from build123d import *

# Parameters (mm, degrees)
SKETCH1_R               = 26.25
BOSS_EXTRUDE1_DEPTH     = 1.5
SKETCH2_R               = 17.5
CUT_EXTRUDE1_DEPTH      = 4.5
SKETCH3_R               = 1
CUT_EXTRUDE2_DEPTH      = 2.5
SKETCH5_R               = 1
CUT_EXTRUDE3_DEPTH      = 1.5
BOSS_EXTRUDE4_DEPTH     = 1.5
CUT_EXTRUDE4_DEPTH      = 10
CUT_EXTRUDE4_DEPTH_BACK = 1.5
SKETCH7_R               = 1.75
SKETCH12_R              = 2.5
BOSS_EXTRUDE6_DEPTH     = 1.5
CUT_EXTRUDE5_START      = 1.5
SKETCH13_R              = 1.75
CUT_EXTRUDE5_DEPTH      = 1.5
BOSS_EXTRUDE8_DEPTH     = 1.5


with BuildPart() as part:
    # Sketch1 → Boss-Extrude1 (new body)
    with BuildSketch(Plane(origin=(0, 0, 0), x_dir=(1, 0, 0), z_dir=(0, 1, 0))):
        with Locations(Location((0, 0, 0), (0, 0, 270))):
            Circle(SKETCH1_R)
    extrude(amount=BOSS_EXTRUDE1_DEPTH)

    # Sketch2 → Cut-Extrude1 (cut)
    with BuildSketch(Plane(origin=(0, 1.5, 0), x_dir=(1, 0, 0), z_dir=(0, 1, 0))):
        with Locations(Location((0, 0, 0), (0, 0, 270))):
            Circle(SKETCH2_R)
    extrude(amount=-CUT_EXTRUDE1_DEPTH, mode=Mode.SUBTRACT)

    # Sketch3 → Cut-Extrude2 (cut)
    with BuildSketch(Plane(origin=(0, 1.5, 0), x_dir=(1, 0, 0), z_dir=(0, 1, 0))):
        with Locations(Location((0, 24.5, 0), (0, 0, 270))):
            Circle(SKETCH3_R)
        with Locations(Location((3.197891709, 24.290399104, 0), (0, 0, 270))):
            Circle(SKETCH3_R)
        with Locations(Location((6.341066605, 23.665182744, 0), (0, 0, 270))):
            Circle(SKETCH3_R)
        with Locations(Location((9.375744093, 22.635048547, 0), (0, 0, 270))):
            Circle(SKETCH3_R)
        with Locations(Location((12.25, 21.217622393, 0), (0, 0, 270))):
            Circle(SKETCH3_R)
        with Locations(Location((14.914655011, 19.437156837, 0), (0, 0, 270))):
            Circle(SKETCH3_R)
        with Locations(Location((17.324116139, 17.324116139, 0), (0, 0, 270))):
            Circle(SKETCH3_R)
        with Locations(Location((19.437156837, 14.914655011, 0), (0, 0, 270))):
            Circle(SKETCH3_R)
        with Locations(Location((21.217622393, 12.25, 0), (0, 0, 270))):
            Circle(SKETCH3_R)
        with Locations(Location((22.635048547, 9.375744093, 0), (0, 0, 270))):
            Circle(SKETCH3_R)
        with Locations(Location((23.665182744, 6.341066605, 0), (0, 0, 270))):
            Circle(SKETCH3_R)
        with Locations(Location((24.290399104, 3.197891709, 0), (0, 0, 270))):
            Circle(SKETCH3_R)
        with Locations(Location((24.5, 0, 0), (0, 0, 270))):
            Circle(SKETCH3_R)
        with Locations(Location((24.290399104, -3.197891709, 0), (0, 0, 270))):
            Circle(SKETCH3_R)
        with Locations(Location((23.665182744, -6.341066605, 0), (0, 0, 270))):
            Circle(SKETCH3_R)
        with Locations(Location((22.635048547, -9.375744093, 0), (0, 0, 270))):
            Circle(SKETCH3_R)
        with Locations(Location((21.217622393, -12.25, 0), (0, 0, 270))):
            Circle(SKETCH3_R)
        with Locations(Location((19.437156837, -14.914655011, 0), (0, 0, 270))):
            Circle(SKETCH3_R)
        with Locations(Location((17.324116139, -17.324116139, 0), (0, 0, 270))):
            Circle(SKETCH3_R)
        with Locations(Location((14.914655011, -19.437156837, 0), (0, 0, 270))):
            Circle(SKETCH3_R)
        with Locations(Location((12.25, -21.217622393, 0), (0, 0, 270))):
            Circle(SKETCH3_R)
        with Locations(Location((9.375744093, -22.635048547, 0), (0, 0, 270))):
            Circle(SKETCH3_R)
        with Locations(Location((6.341066605, -23.665182744, 0), (0, 0, 270))):
            Circle(SKETCH3_R)
        with Locations(Location((3.197891709, -24.290399104, 0), (0, 0, 270))):
            Circle(SKETCH3_R)
        with Locations(Location((0, -24.5, 0), (0, 0, 270))):
            Circle(SKETCH3_R)
        with Locations(Location((-3.197891709, -24.290399104, 0), (0, 0, 270))):
            Circle(SKETCH3_R)
        with Locations(Location((-6.341066605, -23.665182744, 0), (0, 0, 270))):
            Circle(SKETCH3_R)
        with Locations(Location((-9.375744093, -22.635048547, 0), (0, 0, 270))):
            Circle(SKETCH3_R)
        with Locations(Location((-12.25, -21.217622393, 0), (0, 0, 270))):
            Circle(SKETCH3_R)
        with Locations(Location((-14.914655011, -19.437156837, 0), (0, 0, 270))):
            Circle(SKETCH3_R)
        with Locations(Location((-17.324116139, -17.324116139, 0), (0, 0, 270))):
            Circle(SKETCH3_R)
        with Locations(Location((-19.437156837, -14.914655011, 0), (0, 0, 270))):
            Circle(SKETCH3_R)
        with Locations(Location((-21.217622393, -12.25, 0), (0, 0, 270))):
            Circle(SKETCH3_R)
        with Locations(Location((-22.635048547, -9.375744093, 0), (0, 0, 270))):
            Circle(SKETCH3_R)
        with Locations(Location((-23.665182744, -6.341066605, 0), (0, 0, 270))):
            Circle(SKETCH3_R)
        with Locations(Location((-24.290399104, -3.197891709, 0), (0, 0, 270))):
            Circle(SKETCH3_R)
        with Locations(Location((-24.5, 0, 0), (0, 0, 270))):
            Circle(SKETCH3_R)
        with Locations(Location((-24.290399104, 3.197891709, 0), (0, 0, 270))):
            Circle(SKETCH3_R)
        with Locations(Location((-23.665182744, 6.341066605, 0), (0, 0, 270))):
            Circle(SKETCH3_R)
        with Locations(Location((-22.635048547, 9.375744093, 0), (0, 0, 270))):
            Circle(SKETCH3_R)
        with Locations(Location((-21.217622393, 12.25, 0), (0, 0, 270))):
            Circle(SKETCH3_R)
        with Locations(Location((-19.437156837, 14.914655011, 0), (0, 0, 270))):
            Circle(SKETCH3_R)
        with Locations(Location((-17.324116139, 17.324116139, 0), (0, 0, 270))):
            Circle(SKETCH3_R)
        with Locations(Location((-14.914655011, 19.437156837, 0), (0, 0, 270))):
            Circle(SKETCH3_R)
        with Locations(Location((-12.25, 21.217622393, 0), (0, 0, 270))):
            Circle(SKETCH3_R)
        with Locations(Location((-9.375744093, 22.635048547, 0), (0, 0, 270))):
            Circle(SKETCH3_R)
        with Locations(Location((-6.341066605, 23.665182744, 0), (0, 0, 270))):
            Circle(SKETCH3_R)
        with Locations(Location((-3.197891709, 24.290399104, 0), (0, 0, 270))):
            Circle(SKETCH3_R)
    extrude(amount=-CUT_EXTRUDE2_DEPTH, mode=Mode.SUBTRACT)

    # Sketch5 → Cut-Extrude3 (cut)
    with BuildSketch(Plane(origin=(0, 1.5, 0), x_dir=(1, 0, 0), z_dir=(0, 1, 0))):
        with Locations(Location((0, 19.972095444, 0), (0, 0, 270))):
            Circle(SKETCH5_R)
    extrude(amount=-CUT_EXTRUDE3_DEPTH, mode=Mode.SUBTRACT)

    # Sketch6 → Boss-Extrude4 (add)
    with BuildSketch(Plane(origin=(0, 1.5, 0), x_dir=(1, 0, 0), z_dir=(0, 1, 0))):
        with BuildLine():
            Line((-3, 5.5), (-3, 17.24093965))
            Line((-3, 17.24093965), (0, 18.195849362))
            Line((0, 18.195849362), (3, 17.24093965))
            Line((3, 17.24093965), (3, 5.5))
            ThreePointArc((3, 5.5), (3.732233047, 3.732233047), (5.5, 3))
            Line((5.5, 3), (17.24093965, 3))
            Line((17.24093965, 3), (18.195849362, 0))
            Line((18.195849362, 0), (17.24093965, -3))
            Line((17.24093965, -3), (5.5, -3))
            ThreePointArc((5.5, -3), (3.732233047, -3.732233047), (3, -5.5))
            Line((3, -5.5), (3, -17.24093965))
            Line((3, -17.24093965), (0, -18.195849362))
            Line((0, -18.195849362), (-3, -17.24093965))
            Line((-3, -17.24093965), (-3, -5.5))
            ThreePointArc((-3, -5.5), (-3.732233047, -3.732233047), (-5.5, -3))
            Line((-5.5, -3), (-17.24093965, -3))
            Line((-17.24093965, -3), (-18.195849362, 0))
            Line((-18.195849362, 0), (-17.24093965, 3))
            Line((-17.24093965, 3), (-5.5, 3))
            ThreePointArc((-5.5, 3), (-3.732233047, 3.732233047), (-3, 5.5))
        make_face()
    extrude(amount=-BOSS_EXTRUDE4_DEPTH)

    # Sketch7 → Cut-Extrude4 (cut, two sides: drawn at the far end of the back side and taken through both)
    with BuildSketch(Plane(origin=(0, 1.5, 0), x_dir=(1, 0, 0), z_dir=(0, 1, 0)).offset(-CUT_EXTRUDE4_DEPTH_BACK)):
        with Locations(Location((0, 0, 0), (0, 0, 270))):
            Circle(SKETCH7_R)
    extrude(amount=CUT_EXTRUDE4_DEPTH + CUT_EXTRUDE4_DEPTH_BACK, mode=Mode.SUBTRACT)

    # Sketch12 → Boss-Extrude6 (add)
    with BuildSketch(Plane(origin=(0, 1.5, 0), x_dir=(1, 0, 0), z_dir=(0, 1, 0))):
        with Locations(Location((0, 0, 0), (0, 0, 270))):
            Circle(SKETCH12_R)
    extrude(amount=BOSS_EXTRUDE6_DEPTH)

    # Sketch13 → Cut-Extrude5 (cut)
    with BuildSketch(Plane(origin=(0, 1.5, 0), x_dir=(1, 0, 0), z_dir=(0, 1, 0)).offset(CUT_EXTRUDE5_START)):
        with Locations(Location((0, 0, 0), (0, 0, 270))):
            Circle(SKETCH13_R)
    extrude(amount=-CUT_EXTRUDE5_DEPTH, mode=Mode.SUBTRACT)

    # Sketch15 → Boss-Extrude8 (add)
    with BuildSketch(Plane(origin=(0, 1.5, 0), x_dir=(1, 0, 0), z_dir=(0, 1, 0))):
        Polygon((0, 2.35221672), (0, 2.5), (0, 3.865552121), (-0.3804441, 2.470882896), align=None)
        Polygon((0, 3.865552121), (0, 2.5), (0, 2.35221672), (0.3804441, 2.470882896), align=None)
        Polygon((0.763763521, 2.22476713), (0.442463776, 2.460533643), (1.255142722, 3.656105844), (1.162124954, 2.213473648), align=None)
        Polygon((1.444761413, 1.856229501), (1.217423836, 2.18354739), (2.374271254, 3.05046377), (1.817871537, 1.716200185), align=None)
        Polygon((1.969196988, 1.286540603), (1.860457133, 1.669939896), (3.236110655, 2.114256612), (2.276623532, 1.032949802), align=None)
        Polygon((2.280239514, 0.577435067), (2.301881031, 0.975368503), (3.747267254, 0.948936945), (2.488668042, 0.23776328), align=None)
        Polygon((2.344182708, -0.194244517), (2.493860403, 0.175100798), (3.8523493, -0.319214764), (2.431026754, -0.583188583), align=None)
        Polygon((-1.444761413, 1.856229501), (-1.817871537, 1.716200185), (-2.374271254, 3.05046377), (-1.217423836, 2.18354739), align=None)
        Polygon((-1.969196988, 1.286540603), (-2.276623532, 1.032949802), (-3.236110655, 2.114256612), (-1.860457133, 1.669939896), align=None)
        Polygon((-2.280239514, 0.577435067), (-2.488668042, 0.23776328), (-3.747267254, 0.948936945), (-2.301881031, 0.975368503), align=None)
        Polygon((-2.344182708, -0.194244517), (-2.431026754, -0.583188583), (-3.8523493, -0.319214764), (-2.493860403, 0.175100798), align=None)
        Polygon((-2.154097331, -0.944874694), (-2.109945995, -1.340942913), (-3.539969525, -1.552774601), (-2.415591304, -0.644141795), align=None)
        Polygon((-1.730582084, -1.593113037), (-1.560219849, -1.953385272), (-2.843979123, -2.618067215), (-2.075555405, -1.39358163), align=None)
        Polygon((-1.119531416, -2.068712863), (-0.841419673, -2.354148027), (-1.839799454, -3.399651624), (-1.510600873, -1.992005272), align=None)
        Polygon((-0.387162147, -2.32013555), (-0.03143862, -2.499802315), (-0.636248967, -3.812831028), (-0.781949296, -2.374564233), align=None)
        Polygon((1.119531416, -2.068712863), (1.510600873, -1.992005272), (1.839799454, -3.399651624), (0.841419673, -2.354148027), align=None)
        Polygon((1.730582084, -1.593113037), (2.075555405, -1.39358163), (2.843979123, -2.618067215), (1.560219849, -1.953385272), align=None)
        Polygon((2.154097331, -0.944874694), (2.415591304, -0.644141795), (3.539969525, -1.552774601), (2.109945995, -1.340942913), align=None)
        Polygon((-1.162124954, 2.213473648), (-1.255142722, 3.656105844), (-0.442463776, 2.460533643), (-0.763763521, 2.22476713), align=None)
        Polygon((0.781949296, -2.374564233), (0.636248967, -3.812831028), (0.03143862, -2.499802315), (0.387162147, -2.32013555), align=None)
    extrude(amount=BOSS_EXTRUDE8_DEPTH)


solid = part.part
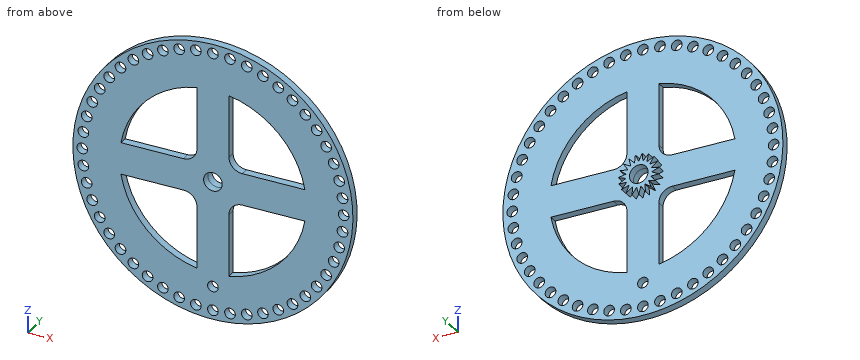
For this review, take the finished solid that the model builds, in its own axes (mm). Round coordinates to 2 decimals unless told otherwise and drop trailing zeros. Write each loop counter-clockwise with the first axis right and the second up, starting at its lowest first coordinate (ties: lowest second). Pieces come first, ordered by that corner, then holes. Notation, with made-up numbers: (20.25, 86.25) -> (27.25, 86.25) arc R38 ccw to (27.25, 124.25) -> close; hole circle Ø6 at (31, 73). An arc over 180 degrees is marked (long way). Put each result on its own line as item: value.
Q1. Consider section B-B on z = 12.25. State the section outline as (x, y) points, and give its area (3 significant figures).
Determined:
outline: (-23.22, 0) -> (-22.22, 0) -> (-22.22, 1.5) -> (-23.22, 1.5) -> close; (-20.22, 0) -> (-12.5, 0) -> (-12.5, 1.5) -> (-20.22, 1.5) -> close; (-3, 0) -> (3, 0) -> (3, 1.5) -> (-3, 1.5) -> close; (12.5, 0) -> (20.22, 0) -> (20.22, 1.5) -> (12.5, 1.5) -> close; (22.22, 0) -> (23.22, 0) -> (23.22, 1.5) -> (22.22, 1.5) -> close
area: 35.2 mm^2
Q2. Consider section A-A on x = -12.25. State the section outline as (y, z) points, and give its area (3 significant figures).
Determined:
outline: (0, -23.22) -> (1.5, -23.22) -> (1.5, -22.22) -> (0, -22.22) -> close; (0, -20.22) -> (1.5, -20.22) -> (1.5, -12.5) -> (0, -12.5) -> close; (0, -3) -> (1.5, -3) -> (1.5, 3) -> (0, 3) -> close; (0, 12.5) -> (1.5, 12.5) -> (1.5, 20.22) -> (0, 20.22) -> close; (0, 22.22) -> (1.5, 22.22) -> (1.5, 23.22) -> (0, 23.22) -> close
area: 35.2 mm^2
Q3. To check wall thickness, follow L1, parallel to X at y = 0.65, z = -22.5; L2, parallel to X at y = 0.35, z = -17.5; L3, parallel to Z at x = -7, y = 0.75. State the ranges of each line that lie inside material, in increasing order. Write a range as [from, to].
Determined:
L1: x = [-13.52, -10.37], [-8.38, 8.38], [10.37, 13.52]
L2: x = [-19.57, -18.31], [-16.34, 16.34], [18.31, 19.57]
L3: z = [-25.3, -24.42], [-22.91, -16.04], [-3, 3], [16.04, 22.91], [24.42, 25.3]
Q4. Clearance check with flat-ended pins moving along their axes: pin 1 Ø4 at (x, z) = (-3, 1.5) entering from +Y; pin 2 Ø2.5 at (x, z) = (23.67, -6.34) entering from +Y; pin 3 Ø1.5 at (y, z) = (2, -10.5) entering from -X; pin 4 Ø1.6 at (x, y) = (9.5, 1) entering from +Z. State where each tip first meets the part, or that it passes through.
Determined:
pin 1: stops at y = 3
pin 2: stops at y = 1.5
pin 3: stops at x = -24.29
pin 4: stops at z = 24.77
Q5. Consider section C-C on y = 0.55. Give the number of separate pieces and of enclosed holes in the cut face, and give its area (3 significant figures).
Determined:
separate pieces: 1
enclosed holes: 54
area: 1,430 mm^2
